Autodesk Inventor part; units mm, degrees
ref_plane "YZ Plane" through (0, 0, 0) normal (1, 0, 0) x (0, 1, 0)
ref_plane "XZ Plane" through (0, 0, 0) normal (0, 1, 0) x (-1, 0, 0)
ref_plane "XY Plane" through (0, 0, 0) normal (0, 0, 1) x (1, 0, 0)
sketch "Szkic1" plane through (0, 0, 0) normal (0, 1, 0) x (-1, 0, 0)
  circle A0 centre (0, 0) radius 5
  dimension "d0" = 10
extrude "Wyciągnięcie proste1" add sketch "Szkic1" along normal blind 8
sketch "Szkic2" plane through (0, 8, 0) normal (0, 1, 0) x (1, 0, 0)
  line L0 (-2.75, -1.5877) -> (-2.75, 1.5877)
  line L1 (-2.75, 1.5877) -> (0, 3.1754)
  line L2 (0, 3.1754) -> (2.75, 1.5877)
  line L3 (2.75, 1.5877) -> (2.75, -1.5877)
  line L4 (2.75, -1.5877) -> (0, -3.1754)
  line L5 (0, -3.1754) -> (-2.75, -1.5877)
  line L6 (0, 7) -> (0, -7)
  point P0 (0, 0)
  point P1 (0, 0)
  dimension "d3" = 5.5
extrude "Wyciągnięcie proste2" cut sketch "Szkic2" against normal blind 3
sketch "Szkic3" plane through (0, 5, 0) normal (0, 1, 0) x (1, 0, 0)
  circle A0 centre (0, 0) radius 5
  circle A1 centre (0, 0) radius 1.25
  dimension "d6" = 2.5
extrude "Wyciągnięcie proste3" cut sketch "Szkic3" against normal through all contours A1
properties part number "housing_legs"
Input: part model. Units: mm. Frame: model coordinates. A direction names the side the tool comes from. Give positions to 0.01 mm unless a question says otherwise; leave off trailing zeros. Loops run counter-clockwise (first coordinate to the right, second up) from the corner with the lowest first, then second, coordinate; pieces in that order, holes last. Notation, with made-up numbers: (65.25, 44.5) -> (92.25, 44.5) arc R27 cw to (92.25, 60.5) -> close; hole circle Ø11 at (-14, 86.5). An arc over 180 degrees is marked (long way). Answer as a JSON object with one key per item and string values. Group by question number.
Item 1: Pin query (flat end, axial travel): P1, Ø1.5, axis at x = -3, z = 1.5, coming from the -Y side; P2, Ø3, axis at x = 0, z = 0, coming from the +Y side; P3, Ø3, axis at y = 3, z = -3, coming from the +X side; P4, Ø3, axis at x = -3.5, y = 3.5, coming from the +Z side. Return the tip coordinate at first contact, or that it passes through.
Item 2: Cut plane C-C, the plane x = 1. Return the cut outline in (y, z), and give its area (3 significant figures).
Item 3: Reachability of faces 4 (the flat face through (-2.75, 7, 0)), 5 (the flat face through (-1, 0, -1)) from +Z, -Z, +X, -X, +Y, -Y: full face, straight path, thin tool, end or side. Return the list, or none.
Item 4: Line query: probe 1 along Z at (x, y) = (0, 3.4); probe 2 along Y at (x, z) = (-1.75, 1); probe 3 along X at (y, z) = (4.5, 0.5). Output: solid intervals per line, ascending.
Item 5: Cut plane A-A, the plane z = 0. Return the cut outline in (x, y), and give its area (3 significant figures).
Item 6: Pull-direction query (Z, two-part tool) for faces 1 (the flat face through (-2.2, 8, -2.2)), 2 (the cylindrical face through (1.08, 3.94, 4.88)), 3 (the flat face through (-1.36, 6.52, 2.39)); classes: released by +Z, released by -Z, zero draft, split by the parting line, or undercut.
Item 7: Cut plane B-B, the plane y = 5.75. Return the cut outline in (x, z).
Item 8: Cut plane D-D, the plane z = -1.75. Return the cut outline in (x, y).
Checks:
{
 "1": {"P1": "stops at y = 0", "P2": "stops at y = 5", "P3": "stops at x = 4.77", "P4": "stops at z = 4.58"},
 "2": {"outline": "(0, -4.9) -> (8, -4.9) -> (8, -2.6) -> (5, -2.6) -> (5, -0.75) -> (0, -0.75) -> close; (0, 0.75) -> (5, 0.75) -> (5, 2.6) -> (8, 2.6) -> (8, 4.9) -> (0, 4.9) -> close", "area": "55.3 mm²"},
 "3": {"face 4": "+Y", "face 5": "+Z, -Z, +X, -X, -Y"},
 "4": {"probe 1": "z = -5 to -1.25, 1.25 to 5", "probe 2": "y = 0 to 5", "probe 3": "x = -4.97 to -1.15, 1.15 to 4.97"},
 "5": {"outline": "(-5, 0) -> (-1.25, 0) -> (-1.25, 5) -> (-2.75, 5) -> (-2.75, 8) -> (-5, 8) -> close; (1.25, 0) -> (5, 0) -> (5, 8) -> (2.75, 8) -> (2.75, 5) -> (1.25, 5) -> close", "area": "51.0 mm²"},
 "6": {"face 1": "zero draft", "face 2": "split by the parting line", "face 3": "undercut"},
 "7": {"outline": "circle Ø10 at (0, 0); hole (-2.75, -1.59) -> (0, -3.18) -> (2.75, -1.59) -> (2.75, 1.59) -> (0, 3.18) -> (-2.75, 1.59) -> close"},
 "8": {"outline": "(-4.68, 0) -> (4.68, 0) -> (4.68, 8) -> (2.47, 8) -> (2.47, 5) -> (-2.47, 5) -> (-2.47, 8) -> (-4.68, 8) -> close"}
}
